Check sheet for the modelled part. Datum: model origin and axes. Units: mm. Face numbers are marked on the shaded views. Round coordinates to 2 decimals unless told otherwise and drop trailing zeros. Loops run counter-clockwise (first coordinate to the right, second up) from the corner with the lowest first, then second, coordinate; pieces in that order, holes last. Notation, with made-up numbers: (53, -9.5) - (62, -9.5) arc R28 ccw to (62, 8.5) - close; hole circle Ø7 at (62.25, -40). An arc over 180 degrees is marked (long way). Put each result on its own line as item: value. Start each with the question number.
Item 1: Section check A-A, the plane x = 85. Record the cut outline in (y, z), and give its area (3 significant figures).
Item 2: Material ranges on line 1 along Z through (x, y) = (85, 1.65); line 2 along X through (y, z) = (0.9, -10); line 3 along Z through (x, y) = (22, 2.85), recorded low to high.
Item 3: Gauge pin test, flat end, axial feed: pin 1 Ø10 at (x, z) = (-17, 28) entering from +Y. Record the tip position at first contact, or that the pin passes through.
Item 4: Draft check along Z on the marked faces 1 and 2. Enter one of: pulls with the +Z half, pulls with the -Z half, needs draft (parallel to the pull), parting line crosses it, or undercut.
Item 5: Section check B-B, the plane y = 3.15. Record the cut outline in (x, z), and give its area (3 significant figures).
Item 6: Section check D-D, the plane z = 40.5. Record the cut outline in (x, y).
Item 7: Section check C-C, the plane x = -46.5. Record the cut outline in (y, z).
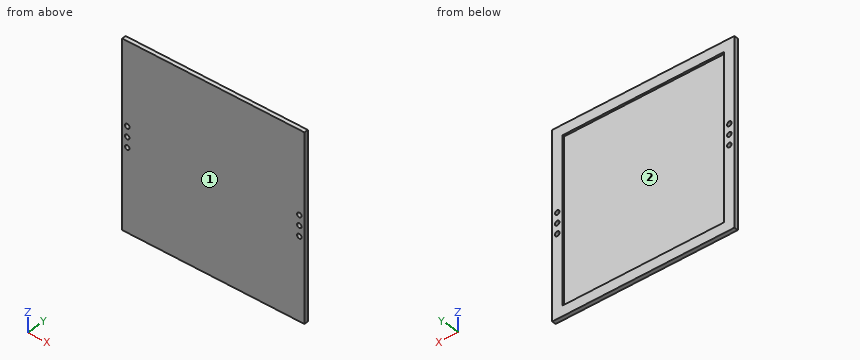
from build123d import *

# Parameters (mm, degrees)
EXTRUDE_1_DEPTH          = 2
EXTRUDE_2_DEPTH          = 4
CUT_EXTRUDE_1_DEPTH      = 128.342059038
CUT_EXTRUDE_1_DEPTH_BACK = 128.342059038
SKETCH_3_R               = 2.25


with BuildPart() as part:
    # Sketch 2 → Extrude 1 (new body)
    with BuildSketch(Plane(origin=(0, 0, 0), x_dir=(1, 0, 0), z_dir=(0, 1, 0))):
        Polygon((-80, 90), (-90, 90), (-90, -90), (90, -90), (90, 90), align=None)
    extrude(amount=EXTRUDE_1_DEPTH)

    # Sketch 2_3 → Extrude 2 (add)
    with BuildSketch(Plane(origin=(0, 0, 0), x_dir=(1, 0, 0), z_dir=(0, 1, 0))):
        Polygon((80, 90), (-80, 90), (-90, 90), (-90, -90), (-80, -90), (90, -90), (90, -80), (90, 90), align=None)
        Polygon((-80, 80), (0, 80), (80, 80), (80, -80), (-80, -80), align=None, mode=Mode.SUBTRACT)
    extrude(amount=EXTRUDE_2_DEPTH)

    # Sketch 3 → Cut-Extrude 1 (cut, two sides: drawn at the far end of the back side and taken through both)
    with BuildSketch(Plane(origin=(0, 4, 0), x_dir=(1, 0, 0), z_dir=(0, 1, 0)).offset(-CUT_EXTRUDE_1_DEPTH_BACK)):
        with BuildLine():
            ThreePointArc((-85, 12.25), (-87.25, 10), (-85, 7.75))
            Line((-85, 7.75), (-85, 10))
            Line((-85, 10), (-85, 12.25))
        make_face()
        with BuildLine():
            Line((-85, 10), (-85, 7.75))
            ThreePointArc((-85, 7.75), (-83.409009742, 8.409009742), (-82.75, 10))
            ThreePointArc((-82.75, 10), (-83.409009742, 11.590990258), (-85, 12.25))
            Line((-85, 12.25), (-85, 10))
        make_face()
        with BuildLine():
            ThreePointArc((-85, -2.25), (-83.409009742, -1.590990258), (-82.75, 0))
            Line((-82.75, 0), (-85, 0))
            Line((-85, 0), (-85, -2.25))
        make_face()
        with BuildLine():
            Line((-85, 0), (-82.75, 0))
            ThreePointArc((-82.75, 0), (-83.409009742, 1.590990258), (-85, 2.25))
            Line((-85, 2.25), (-85, 0))
        make_face()
        with BuildLine():
            Line((-85, -2.25), (-85, 0))
            Line((-85, 0), (-87.25, 0))
            ThreePointArc((-87.25, 0), (-86.590990258, -1.590990258), (-85, -2.25))
        make_face()
        with BuildLine():
            Line((-87.25, 0), (-85, 0))
            Line((-85, 0), (-85, 2.25))
            ThreePointArc((-85, 2.25), (-86.590990258, 1.590990258), (-87.25, 0))
        make_face()
        with BuildLine():
            ThreePointArc((-82.75, -10), (-83.409009742, -8.409009742), (-85, -7.75))
            Line((-85, -7.75), (-85, -10))
            Line((-85, -10), (-85, -12.25))
            ThreePointArc((-85, -12.25), (-83.409009742, -11.590990258), (-82.75, -10))
        make_face()
        with BuildLine():
            Line((-85, -10), (-85, -7.75))
            ThreePointArc((-85, -7.75), (-87.25, -10), (-85, -12.25))
            Line((-85, -12.25), (-85, -10))
        make_face()
        with Locations(Location((85, 10, 0), (0, 0, 270))):
            Circle(SKETCH_3_R)
        with BuildLine():
            ThreePointArc((87.25, 0), (85, 2.25), (82.75, 0))
            Line((82.75, 0), (87.25, 0))
        make_face()
        with BuildLine():
            Line((87.25, 0), (82.75, 0))
            ThreePointArc((82.75, 0), (85, -2.25), (87.25, 0))
        make_face()
        with Locations(Location((85, -10, 0), (0, 0, 270))):
            Circle(SKETCH_3_R)
    extrude(amount=CUT_EXTRUDE_1_DEPTH + CUT_EXTRUDE_1_DEPTH_BACK, mode=Mode.SUBTRACT)


solid = part.part
Check result:
1. outline: (0, -90) - (4, -90) - (4, -12.25) - (0, -12.25) - close; (0, -7.75) - (4, -7.75) - (4, -2.25) - (0, -2.25) - close; (0, 2.25) - (4, 2.25) - (4, 7.75) - (0, 7.75) - close; (0, 12.25) - (4, 12.25) - (4, 90) - (0, 90) - close
1. area: 666 mm²
2. line 1: -90 to -12.25, -7.75 to -2.25, 2.25 to 7.75, 12.25 to 90
2. line 2: -90 to -87.25, -82.75 to 82.75, 87.25 to 90
2. line 3: -90 to -80, 80 to 90
3. pin 1: y = 2
4. face 1: needs draft
4. face 2: undercut
5. outline: (-90, -90) - (90, -90) - (90, 90) - (-90, 90) - close; hole circle Ø4.5 at (-85, -10); hole circle Ø4.5 at (-85, 0); hole circle Ø4.5 at (-85, 10); hole (-80, -80) - (80, -80) - (80, 80) - (-80, 80) - close; hole circle Ø4.5 at (85, -10); hole circle Ø4.5 at (85, 0); hole circle Ø4.5 at (85, 10)
5. area: 6,700 mm²
6. outline: (-90, 0) - (90, 0) - (90, 4) - (80, 4) - (80, 2) - (-80, 2) - (-80, 4) - (-90, 4) - close
7. outline: (0, -90) - (4, -90) - (4, -80) - (2, -80) - (2, 80) - (4, 80) - (4, 90) - (0, 90) - close
